Verification items for the finished model (mm, model axes). A direction names the side the tool comes from. Give positions to 0.01 mm unless a question says otherwise; leave off trailing zeros. Write each loop counter-clockwise with the first axis right and the second up, starting at its lowest first coordinate (ties: lowest second). Pieces come first, ordered by that corner, then holes. Notation, with made-up numbers: (-25, -28.5) -> (17, -28.5) arc R26 ccw to (17, 9.5) -> close; hole circle Ø1 at (76.25, 61.25). An arc over 180 degrees is marked (long way). Use CSV: the item, a comma, the result in double quotes. Start each with the question number.
```python
from build123d import *

# Parameters (mm, degrees)
ESQUISSE1_R      = 1.6
EXTRUSION1_DEPTH = 2.5
ESQUISSE2_W      = 6.4
ESQUISSE2_H      = 4.7
EXTRUSION2_DEPTH = 8.8
EXTRUSION3_DEPTH = 4.8


with BuildPart() as part:
    # Esquisse1 → Extrusion1 (new body)
    with BuildSketch(Plane(origin=(0, 0, 0), x_dir=(1, 0, 0), z_dir=(0, 1, 0))):
        with BuildLine():
            Line((-3.2, 6.2), (3.2, 6.2))
            Line((3.2, 6.2), (3.2, -9.2))
            ThreePointArc((3.2, -9.2), (0, -12.4), (-3.2, -9.2))
            Line((-3.2, -9.2), (-3.2, 6.2))
        make_face()
        with Locations(Location((0, -9.2, 0), (0, 0, 270))):
            Circle(ESQUISSE1_R, mode=Mode.SUBTRACT)
    extrude(amount=-EXTRUSION1_DEPTH)

    # Esquisse2 → Extrusion2 (add)
    with BuildSketch(Plane(origin=(0, 0, 0), x_dir=(-1, 0, 0), z_dir=(0, 1, 0))):
        with Locations((0, -3.85)):
            Rectangle(ESQUISSE2_W, ESQUISSE2_H)
        with Locations((0, 3.85)):
            Rectangle(ESQUISSE2_W, ESQUISSE2_H)
    extrude(amount=EXTRUSION2_DEPTH)

    # Esquisse3 → Extrusion3 (add)
    with BuildSketch(Plane.XZ.offset(2.5)):
        with BuildLine():
            Line((-2, 3.8), (2, 3.8))
            ThreePointArc((2, 3.8), (2.353553391, 3.653553391), (2.5, 3.3))
            Line((2.5, 3.3), (2.5, 2))
            ThreePointArc((2.5, 2), (2.353553391, 1.646446609), (2, 1.5))
            Line((2, 1.5), (-2, 1.5))
            ThreePointArc((-2, 1.5), (-2.353553391, 1.646446609), (-2.5, 2))
            Line((-2.5, 2), (-2.5, 3.3))
            ThreePointArc((-2.5, 3.3), (-2.353553391, 3.653553391), (-2, 3.8))
        make_face()
        with BuildLine():
            Line((-2, -1.5), (2, -1.5))
            ThreePointArc((2, -1.5), (2.353553391, -1.646446609), (2.5, -2))
            Line((2.5, -2), (2.5, -3.3))
            ThreePointArc((2.5, -3.3), (2.353553391, -3.653553391), (2, -3.8))
            Line((2, -3.8), (-2, -3.8))
            ThreePointArc((-2, -3.8), (-2.353553391, -3.653553391), (-2.5, -3.3))
            Line((-2.5, -3.3), (-2.5, -2))
            ThreePointArc((-2.5, -2), (-2.353553391, -1.646446609), (-2, -1.5))
        make_face()
    extrude(amount=EXTRUSION3_DEPTH)


solid = part.part
```
(1) Go/stop test with flat-tipped pins: pin 1 (3 mm diameter, centred on x = 1, y = 4, fed in from +Z); pin 2 (0.6 mm diameter, centred on y = -5, z = -2.5, fed in from +X); pin 3 (1.4 mm diameter, centred on y = -4, z = -2.5, fed in from -X). Record where each tip stops, or that it passes through.
(2) Section check D-D on y = 3.25. Record the cut outline in (x, z), then the cut area to 3 significant figures.
(3) Set-up check for faces 4 (the face through (0, -5, -3.8)), 5 (the face through (2.5, -5, -3)), 6 (the face through (0, 4, 6.2)): record each of +Z, -Z, +X, -X, +Y, -Y from which the full face is reachable in a straight line by a thin tool's end or side.
(4) Thickness scan on line 1 (X direction, y = -0.45, z = 9.2); line 2 (Z direction, x = 0, y = 8.25); line 3 (Y direction, x = -2.5, z = 5.25). Record the ranges inside material, lowest first. Write a range as from..to.
(5) Draft check along X on faces 1 (the face through (2.5, -5, 3)), 2 (the face through (0.481, -1.232, 10.726)), 3 (the face through (0, -5, 3.8)). Enter one of: released by +X, released by -X, zero draft, split by the parting line, or undercut.
(6) Section check C-C on y = -1.5. Record the cut outline in (x, z).
(7) Section check A-A on y = -5.5. Record the cut outline in (x, z), then the cut area to 3 significant figures.
(8) Section check B-B on x = 0. Record the cut outline in (y, z), then the cut area to 3 significant figures.
Data:
1,pin 1,"stops at z = 6.2"
1,pin 2,"stops at x = 2.5"
1,pin 3,"stops at x = -2.5"
2,outline,"(-3.2, -6.2) -> (3.2, -6.2) -> (3.2, -1.5) -> (-3.2, -1.5) -> close; (-3.2, 1.5) -> (3.2, 1.5) -> (3.2, 6.2) -> (-3.2, 6.2) -> close"
2,area,"60.2 mm2"
3,face 4,"-Z, +X, -X, -Y"
3,face 5,"+Z, -Z, +X, -Y"
3,face 6,"+Z, +X, -X, +Y"
4,line 1,"x = -3.2..-1.6, 1.6..3.2"
4,line 2,"z = -6.2..-1.5, 1.5..6.2"
4,line 3,"y = -2.5..8.8"
5,face 1,"released by +X"
5,face 2,"undercut"
5,face 3,"zero draft"
6,outline,"(-3.2, -6.2) -> (3.2, -6.2) -> (3.2, 9.2) arc R3.2 ccw to (-3.2, 9.2) -> close; hole circle Ø3.2 at (0, 9.2)"
7,outline,"(-2.5, -3.3) arc R0.5 ccw to (-2, -3.8) -> (2, -3.8) arc R0.5 ccw to (2.5, -3.3) -> (2.5, -2) arc R0.5 ccw to (2, -1.5) -> (-2, -1.5) arc R0.5 ccw to (-2.5, -2) -> close; (-2.5, 2) arc R0.5 ccw to (-2, 1.5) -> (2, 1.5) arc R0.5 ccw to (2.5, 2) -> (2.5, 3.3) arc R0.5 ccw to (2, 3.8) -> (-2, 3.8) arc R0.5 ccw to (-2.5, 3.3) -> close"
7,area,"22.6 mm2"
8,outline,"(-7.3, -3.8) -> (-2.5, -3.8) -> (-2.5, -6.2) -> (8.8, -6.2) -> (8.8, -1.5) -> (0, -1.5) -> (0, 1.5) -> (8.8, 1.5) -> (8.8, 6.2) -> (0, 6.2) -> (0, 7.6) -> (-2.5, 7.6) -> (-2.5, 3.8) -> (-7.3, 3.8) -> (-7.3, 1.5) -> (-2.5, 1.5) -> (-2.5, -1.5) -> (-7.3, -1.5) -> close; (-2.5, 10.8) -> (0, 10.8) -> (0, 12.4) -> (-2.5, 12.4) -> close"
8,area,"143 mm2"
